Could you check a few things on this model? Use its own coordinates, in mm. A direction names the side the tool comes from. Coordinates: 2 decimals unless noted, no trailing zeros. Write each loop counter-clockwise with the first axis right and the second up, starting at its lowest first coordinate (ties: lowest second). Pieces come first, ordered by that corner, then holes.
Autodesk Fusion 360 part; units mm, degrees
sketch "Skizze1" plane through (0, 0, 0) normal (0, 0, 1) x (1, 0, 0)
  line L0 (-87.8679, 0) -> (-212.132, 0)
  line L1 (-300, -87.868) -> (-300, -212.132)
  line L2 (-212.132, -300) -> (-87.8679, -300)
  line L3 (0, -212.1321) -> (0, -87.8679)
  line L4 (0, -87.8679) -> (-87.8679, 0)
  line L5 (-212.132, 0) -> (-300, -87.868)
  line L6 (-300, -212.132) -> (-212.132, -300)
  line L7 (-87.8679, -300) -> (0, -212.1321)
  dimension "d3" = 45
  dimension "d4" = 45
  dimension "d5" = 300
  dimension "d6" = 300
  dimension "d9" = 87.8679
  dimension "d10" = 87.8679
  dimension "d11" = 300
  dimension "d12" = 300
extrude "Extrusion1" add sketch "Skizze1" along normal blind 18
sketch "Skizze2" plane through (0, 0, 18) normal (0, 0, 1) x (-1, 0, 0)
  line L0 (87.8679, 300) -> (0, 212.1321)
  line L1 (0, 212.1321) -> (0, 87.8679)
  line L2 (0, 87.8679) -> (87.8679, 0)
  line L3 (87.8679, 0) -> (212.132, 0)
  line L4 (212.132, 0) -> (300, 87.868)
  line L5 (300, 87.868) -> (300, 212.132)
  line L6 (300, 212.132) -> (212.132, 300)
  line L7 (212.132, 300) -> (87.8679, 300)
  circle A0 centre (150, 150) radius 110
  dimension "d15" = 150
  dimension "d16" = 150
  dimension "d17" = 220
extrude "Extrusion2" cut sketch "Skizze2" against normal blind 18 contours A0
sketch "Skizze3" plane through (0, 0, 0) normal (0, 0, -1) x (1, 0, 0)
  circle A0 centre (-150, 150) radius 110
  line L0 (0, 212.1321) -> (-87.8679, 300)
  line L1 (-87.8679, 300) -> (-212.132, 300)
  line L2 (-212.132, 300) -> (-300, 212.132)
  line L3 (-300, 212.132) -> (-300, 87.868)
  line L4 (-300, 87.868) -> (-212.132, 0)
  line L5 (-212.132, 0) -> (-87.8679, 0)
  line L6 (-87.8679, 0) -> (0, 87.8679)
  line L7 (0, 87.8679) -> (0, 212.1321)
  line L8 (-65.2405, 90.5097) -> (-51.0983, 76.3675)
  line L9 (-51.0983, 76.3675) -> (-79.3826, 48.0833)
  line L10 (-79.3826, 48.0833) -> (-93.5248, 62.2254)
  line L11 (-93.5248, 62.2254) -> (-65.2405, 90.5097)
  dimension "d20" = 28
  dimension "d21" = 40
  dimension "d22" = 40
  dimension "d23" = 20
extrude "Extrusion3" cut sketch "Skizze3" against normal blind 10 contours A0 L8 L9 L10
sketch "Skizze4" plane through (0, 0, 0) normal (0, 1, 0) x (-1, 0, 0)
  line L0 (87.8679, 0) -> (212.132, 0)
  line L1 (212.132, 0) -> (212.132, 18)
  line L2 (212.132, 18) -> (87.8679, 18)
  line L3 (87.8679, 18) -> (87.8679, 0)
  line L4 (144.8679, 6.5) -> (154.8679, 6.5)
  arc A0 (154.8679, 6.5) -> (154.8679, 11.5) centre (154.8679, 9) ccw
  line L5 (154.8679, 11.5) -> (144.8679, 11.5)
  arc A1 (144.8679, 11.5) -> (144.8679, 6.5) centre (144.8679, 9) ccw
  dimension "d26" = 5
  dimension "d27" = 10
  dimension "d28" = 9
  dimension "d30" = 57
extrude "Extrusion4" cut sketch "Skizze4" against normal blind 20 contours L4 A0 L5 A1
sketch "Skizze5" plane through (0, -20, 0) normal (0, 1, 0) x (-1, 0, 0)
  arc A0 (144.8679, 11.5) -> (144.8679, 6.5) centre (144.8679, 9) ccw
  line L0 (144.8679, 6.5) -> (154.8679, 6.5)
  arc A1 (154.8679, 6.5) -> (154.8679, 11.5) centre (154.8679, 9) ccw
  line L1 (154.8679, 11.5) -> (144.8679, 11.5)
  circle A2 centre (149.8679, 9) radius 2.5
  dimension "d33" = 5
  dimension "d34" = 5
  dimension "d35" = 2.5
extrude "Extrusion5" cut sketch "Skizze5" against normal blind 40 contours A2
equation "d30 = ( 124 / 2 ) * 1 mm - 5 mm"
1. On a 3-axis mill with a long thin cutter (end or side, diameter ignored), from which of +Z, -Z, +X, -X, +Y, -Y can I reach the whole of each face in a straight line? I mean faces 1 (the face through (-43.32, -44.55, 8.87)), 2 (the face through (-84.4, -53.1, 4.9)), 3 (the face through (-150, -10, 6.5)). Say none if no direction works.
Verdict:
face 1: +Z, -Z, +X, +Y
face 2: -Z
face 3: +Y
2. I want a section at B-B on x = -186. Please give me the cut outline in (y, z), plus the area to 3 significant figures.
Verdict:
outline: (-300, 0) - (-253.94, 0) - (-253.94, 18) - (-300, 18) - close; (-46.06, 0) - (0, 0) - (0, 18) - (-46.06, 18) - close
area: 1,660 mm2
3. I want a section at A-A on y = -150. Please give me the cut outline in (x, z).
Verdict:
outline: (-300, 0) - (-260, 0) - (-260, 18) - (-300, 18) - close; (-40, 0) - (0, 0) - (0, 18) - (-40, 18) - close
4. Please list where these lines run through material, in increasing order: line 1 along Y through (x, z) = (-150, 14); line 2 along Y through (x, z) = (-55, 6.25).
Verdict:
line 1: y = -300 to -260, -40 to 0
line 2: y = -267.13 to -205.45, -94.55 to -80.27, -72.47 to -32.87
5. For pin 1 (4 mm diameter, centred on x = -149.87, z = 9, fed in from +Y); pin 2 (10 mm diameter, centred on y = -229, z = 11.5, fed in from +X); pin 3 (2 mm diameter, centred on x = -263.5, z = 11.5, fed in from -Y), each with a flat end and sliding along its axis, tell me the tip position at first contact or that it passes through.
Verdict:
pin 1: stops at y = -259.98
pin 2: stops at x = -11.87
pin 3: stops at y = -249.63
6. If we mould it in two halves opening along X, with no side actions, what happens to faces 4 (the face through (-209.14, -242.75, 9.13)), 5 (the face through (-300, -149, 9)), 6 (the face through (-52, -215, 18))? For each: pulls with the +X half, pulls with the -X half, needs draft (parallel to the pull), parting line crosses it, or undercut.
Verdict:
face 4: undercut
face 5: pulls with the -X half
face 6: needs draft
